from build123d import *

# Parameters (mm, degrees)
SKETCH1_W           = 36
SKETCH1_H           = 107
BOSS_EXTRUDE1_DEPTH = 28
FILLET1_R           = 10


with BuildPart() as part:
    # Sketch1 → Boss-Extrude1 (new body)
    with BuildSketch(Plane(origin=(0, 0, 0), x_dir=(1, 0, 0), z_dir=(0, 1, 0))):
        with Locations((18, 53.5)):
            Rectangle(SKETCH1_W, SKETCH1_H)
    extrude(amount=BOSS_EXTRUDE1_DEPTH)

    # Fillet1
    fillet1_edges = [part.edges().sort_by_distance(p)[0] for p in [
        (36, 28, -53.5),
        (18, 28, -107),
        (0, 28, -53.5),
        (18, 0, -107),
        (36, 0, -53.5),
        (18, 0, 0),
        (0, 0, -53.5),
        (18, 28, 0),
        (36, 14, -107),
    ]]
    fillet(fillet1_edges, radius=FILLET1_R)


solid = part.part
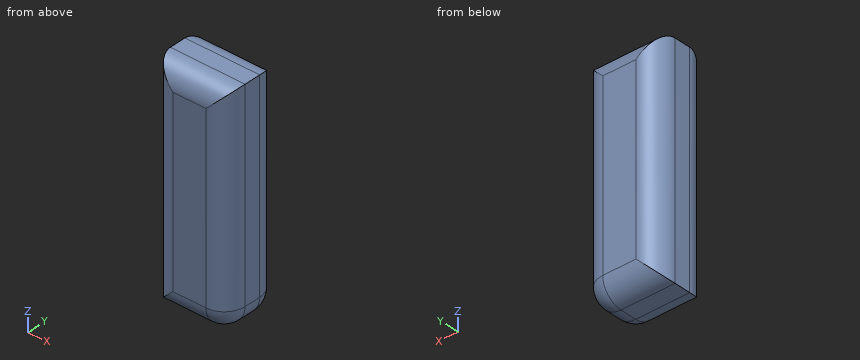
Design review of the part built by this model. Coordinates are the model's own, in mm. Round coordinates to 2 decimals unless told otherwise and drop trailing zeros. Write each loop counter-clockwise with the first axis right and the second up, starting at its lowest first coordinate (ties: lowest second). Pieces come first, ordered by that corner, then holes. Notation, with made-up numbers: (-26, 40.5) - (22, 40.5) arc R21 ccw to (22, 55.5) - close; hole circle Ø1 at (52, -36). An arc over 180 degrees is marked (long way). Return JSON: item names as keys, results as strings. Group by question number.
Item 1: We need section C-C on y = 8. Write out the cut boundary in (x, z).
Item 2: We need section A-A on x = 13. Write out the cut boundary in (y, z).
Item 3: We need section B-B on z = -28. Write out the cut boundary in (x, y).
Item 4: Insertion check: P1, Ø1, axis at x = 7, y = 23.5, coming from the -Z side; P2, Ø6, axis at y = 22.5, z = -59, coming from the +X side. Each pin has a flat end and moves straight along its axis. Give the tip position at first contact, or say it passes through.
Item 5: For probe 1 along Z at (x, y) = (26.5, 12.5); probe 2 along X at (y, z) = (8.25, -10); probe 3 along X at (y, z) = (6, -64.5), list the stretches that pass through material, from the lowest coordinate up. Write a range as [from, to].
Item 6: We need section D-D on y = 3.25. Write out the cut boundary in (x, z).
Model answer:
{
 "1": {"outline": "(0.2, -106.8) - (26, -106.8) arc R9.8 ccw to (35.8, -97) - (35.8, -0.2) - (0.2, -0.2) - close"},
 "2": {"outline": "(0, -97) arc R10 ccw to (10, -107) - (18, -107) arc R10 ccw to (28, -97) - (28, -10) arc R10 ccw to (18, 0) - (10, 0) arc R10 ccw to (0, -10) - close"},
 "3": {"outline": "(0, 10) arc R10 ccw to (10, 0) - (26, 0) arc R10 ccw to (36, 10) - (36, 18) arc R10 ccw to (26, 28) - (10, 28) arc R10 ccw to (0, 18) - close"},
 "4": {"P1": "stops at z = -105.66", "P2": "stops at x = 35.89"},
 "5": {"probe 1": "z = [-106.99, 0]", "probe 2": "x = [0.15, 35.85]", "probe 3": "x = [0.83, 35.17]"},
 "6": {"outline": "(2.62, -104.38) - (26, -104.38) arc R7.38 ccw to (33.38, -97) - (33.38, -2.62) - (2.62, -2.62) - close"}
}
